The model under review builds one solid part; all positions refer to its coordinate system, in mm. A direction names the side the tool comes from. Give positions to 0.01 mm unless a question says otherwise; leave off trailing zeros. Order: outer loops, then holes, each group sorted by start corner. A loop starts at its lowest first (then second) coordinate and runs counter-clockwise, first axis right, second up.
```python
from build123d import *

# Parameters (mm, degrees)
SKETCH1_W             = 25.4
SKETCH1_H             = 101.6
TOP_DEPTH             = 4.7625
SKETCH2_W             = 25.4
SKETCH2_H             = 101.6
SKETCH2_W_2           = 15.875
SKETCH2_H_2           = 88.9
WALLS_DEPTH           = 31.75
SKETCH9_R             = 3.302
JOINT_HINGE_DEPTH     = 6.35
SKETCH3_R             = 3.175
SHAFT_HOLES_DEPTH     = 23.876
SKETCH13_W            = 1.778
SKETCH13_H            = 5.08
WIRE_LOFT_MOUNT_DEPTH = 12.7
ANTI_FLEX_DEPTH       = 3.175
FILLET1_R             = 2.54
FILLET2_R             = 1.5875


with BuildPart() as part:
    # Sketch1 → Top (new body)
    with BuildSketch(Plane(origin=(0, 0, 0), x_dir=(1, 0, 0), z_dir=(0, 1, 0))):
        Rectangle(SKETCH1_W, SKETCH1_H)
    extrude(amount=TOP_DEPTH)

    # Sketch2 → Walls (add)
    with BuildSketch(Plane(origin=(0, 4.7625, 0), x_dir=(1, 0, 0), z_dir=(0, 1, 0))):
        Rectangle(SKETCH2_W, SKETCH2_H)
        Rectangle(SKETCH2_W_2, SKETCH2_H_2, mode=Mode.SUBTRACT)
    extrude(amount=-WALLS_DEPTH)

    # Sketch9 → Joint Hinge (add)
    with BuildSketch(Plane(origin=(0, 0, 50.8), x_dir=(-1, 0, 0), z_dir=(0, 0, -1))):
        with BuildLine():
            Line((-28.956, 4.7625), (-12.7, 4.7625))
            Line((-12.7, 4.7625), (-12.7, -26.9875))
            Line((-12.7, -26.9875), (-14.756968343, -26.9875))
            ThreePointArc((-14.756968343, -26.9875), (-46.346191201, -22.064629933), (-28.956, 4.7625))
        make_face()
        with Locations((-28.956, -14.2875)):
            Circle(SKETCH9_R, mode=Mode.SUBTRACT)
    extrude(amount=JOINT_HINGE_DEPTH)

    # Sketch3 → Shaft holes (cut)
    with BuildSketch(Plane.ZY.offset(12.7)):
        with Locations((38.1, -11.1125)):
            Circle(SKETCH3_R)
        with BuildLine():
            Line((-25.601638938, -12.7), (-23.061638938, -12.7))
            Line((-23.061638938, -12.7), (-23.061638938, -9.525))
            Line((-23.061638938, -9.525), (-25.601638938, -9.525))
            ThreePointArc((-25.601638938, -9.525), (-38.1, -11.1125), (-25.601638938, -12.7))
        make_face()
    extrude(amount=-SHAFT_HOLES_DEPTH, mode=Mode.SUBTRACT)

    # Sketch13 → Wire Loft Mount (cut)
    with BuildSketch(Plane.XZ):
        with Locations((-2.286, 29.21)):
            Rectangle(SKETCH13_W, SKETCH13_H)
    extrude(amount=-WIRE_LOFT_MOUNT_DEPTH, mode=Mode.SUBTRACT)

    # Sketch15 → Anti-flex (add)
    with BuildSketch(Plane(origin=(0, 4.7625, 0), x_dir=(1, 0, 0), z_dir=(0, 1, 0))):
        Polygon((12.7, -44.45), (28.956, -44.45), (12.7, -28.194), align=None)
        Polygon((12.7, 28.194), (28.956, 44.45), (28.956, 50.8), (12.7, 50.8), align=None)
    extrude(amount=-ANTI_FLEX_DEPTH)

    # Fillet1
    fillet1_edges = [part.edges().sort_by_distance(p)[0] for p in [
        (8.128, 4.7625, -50.8),
        (0, -26.9875, -50.8),
        (1.028484171, -26.9875, 50.8),
        (46.346191201, -22.064629933, 50.8),
        (8.128, 4.7625, 50.8),
    ]]
    fillet(fillet1_edges, radius=FILLET1_R)

    # Fillet2
    # the kernel refuses this fillet: 1.5875 mm, written as the material it takes off along each edge
    with BuildSketch(Plane(origin=(9.893669962, 1.5875, -25.387669962), x_dir=(-0.7071067811865515, 0, -0.7071067811865436), z_dir=(0.7071067811865437, 0, -0.7071067811865515))) as fillet2_piece_1_section:
        with BuildLine():
            CenterArc((FILLET2_R, FILLET2_R), FILLET2_R, 180, 90)
            Line((0, FILLET2_R), (0, 0))
            Line((0, 0), (FILLET2_R, 0))
        make_face()
    fillet2_piece_1 = extrude(amount=30.92695567, mode=Mode.PRIVATE)
    fillet2_piece_1 = split(fillet2_piece_1, bisect_by=Plane(origin=(12.7, 1.942096603, -36.823475324), z_dir=(1, 0, 0)), keep=Keep.TOP, mode=Mode.PRIVATE)
    add(fillet2_piece_1, mode=Mode.SUBTRACT)
    with BuildSketch(Plane(origin=(9.893669962, 4.7625, -25.387669962), x_dir=(-0.7071067811865515, 0, -0.7071067811865436), z_dir=(0.7071067811865437, 0, -0.7071067811865515))) as fillet2_piece_2_section:
        with BuildLine():
            CenterArc((FILLET2_R, -FILLET2_R), FILLET2_R, 90, 90)
            Line((0, -FILLET2_R), (0, 0))
            Line((0, 0), (FILLET2_R, 0))
        make_face()
    fillet2_piece_2 = extrude(amount=30.92695567, mode=Mode.PRIVATE)
    fillet2_piece_2 = split(fillet2_piece_2, bisect_by=Plane(origin=(12.7, 4.407903397, -36.823475324), z_dir=(1, 0, 0)), keep=Keep.TOP, mode=Mode.PRIVATE)
    add(fillet2_piece_2, mode=Mode.SUBTRACT)
    with BuildSketch(Plane(origin=(31.762330038, 1.5875, 47.256330038), x_dir=(-0.7071067811865436, 0, 0.7071067811865515), z_dir=(-0.7071067811865515, 0, -0.7071067811865436))) as fillet2_piece_3_section:
        with BuildLine():
            CenterArc((FILLET2_R, FILLET2_R), FILLET2_R, 180, 90)
            Line((0, FILLET2_R), (0, 0))
            Line((0, 0), (FILLET2_R, 0))
        make_face()
    fillet2_piece_3 = extrude(amount=30.92695567, mode=Mode.PRIVATE)
    fillet2_piece_3 = split(fillet2_piece_3, bisect_by=Plane(origin=(12.7, 1.946775649, 36.567113542), z_dir=(1, 0, 0)), keep=Keep.TOP, mode=Mode.PRIVATE)
    fillet2_piece_3 = split(fillet2_piece_3, bisect_by=Plane(origin=(20.582886458, 1.946775649, 44.45), z_dir=(0, 0, -1)), keep=Keep.TOP, mode=Mode.PRIVATE)
    add(fillet2_piece_3, mode=Mode.SUBTRACT)
    with BuildSketch(Plane(origin=(31.762330038, 4.7625, 47.256330038), x_dir=(-0.7071067811865436, 0, 0.7071067811865515), z_dir=(-0.7071067811865515, 0, -0.7071067811865436))) as fillet2_piece_4_section:
        with BuildLine():
            CenterArc((FILLET2_R, -FILLET2_R), FILLET2_R, 90, 90)
            Line((0, -FILLET2_R), (0, 0))
            Line((0, 0), (FILLET2_R, 0))
        make_face()
    fillet2_piece_4 = extrude(amount=30.92695567, mode=Mode.PRIVATE)
    fillet2_piece_4 = split(fillet2_piece_4, bisect_by=Plane(origin=(12.7, 4.227310256, 42.469450936), z_dir=(1, 0, 0)), keep=Keep.TOP, mode=Mode.PRIVATE)
    fillet2_piece_4 = split(fillet2_piece_4, bisect_by=Plane(origin=(26.668449599, 4.227310256, 44.45), z_dir=(0, 0, -1)), keep=Keep.TOP, mode=Mode.PRIVATE)
    add(fillet2_piece_4, mode=Mode.SUBTRACT)
    with BuildSketch(Plane(origin=(31.762330038, 4.7625, 47.256330038), x_dir=(-0.7071067811865436, 0, 0.7071067811865515), z_dir=(-0.7071067811865515, 0, -0.7071067811865436))) as fillet2_piece_5_section:
        with BuildLine():
            CenterArc((FILLET2_R, -FILLET2_R), FILLET2_R, 90, 90)
            Line((0, -FILLET2_R), (0, 0))
            Line((0, 0), (FILLET2_R, 0))
        make_face()
    fillet2_piece_5 = extrude(amount=30.92695567, mode=Mode.PRIVATE)
    fillet2_piece_5 = split(fillet2_piece_5, bisect_by=Plane(origin=(27.86835314, 4.749091996, 44.45), z_dir=(0, 0, 1)), keep=Keep.TOP, mode=Mode.PRIVATE)
    fillet2_piece_5 = fillet2_piece_5 - Plane(origin=(28.956, -14.2875, 44.898632057), x_dir=(-0.7453559924999297, -0.6666666666666669, 0), z_dir=(0, 0, 1)) * Cylinder(19.05, 69, mode=Mode.PRIVATE)
    add(fillet2_piece_5, mode=Mode.SUBTRACT)


solid = part.part
```
Item 1: For line 1 (X direction, y = -23, z = -6.5); line 2 (Y direction, x = -10, z = 38); line 3 (Y direction, x = 16, z = -36.5), list the stretches that pass through material, from the lowest coordinate up.
Values found:
line 1: x = -12.7 to -7.94, 7.94 to 12.7
line 2: y = -26.99 to -14.29, -7.94 to 4.76
line 3: y = 1.59 to 4.76
Item 2: Take a section at A-A (z = 13.5). Give the boundary of the cut face in (x, y), and give its area (3 significant figures).
Values found:
outline: (-12.7, -26.99) - (-7.94, -26.99) - (-7.94, 0) - (7.94, 0) - (7.94, -26.99) - (12.7, -26.99) - (12.7, 4.76) - (-12.7, 4.76) - close
area: 378 mm2
Item 3: Take a section at B-B (x = 9.5). Give the number of separate pieces and of enclosed holes in the cut face, and give its area (3 significant figures).
Values found:
separate pieces: 1
enclosed holes: 2
area: 3,050 mm2
Item 4: Draft analysis for pull direction X (two halves, no side actions). For faces 1 (the flat face through (28.956, 3, -48)), 2 (the cylindrical face through (1.8, -26.3, 50)), 3 (the flat face through (0, -13, -44.45)), state which applies: released by +X, released by -X, zero draft, split by the parting line, or undercut.
Values found:
face 1: released by +X
face 2: zero draft
face 3: undercut
Item 5: For faces 4 (the flat face through (10, -9.525, -24)), 5 (the flat face through (0, -13, 44.45)), 6 (the flat face through (-3.175, 2, 29)), list the 3-axis set-ups (+Z, -Z, +X, -X, +Y, -Y) from which the entire face can be reached by the end or side of a thin tool; tool diameter is ignored.
Values found:
face 4: -X
face 5: -Y
face 6: +Y, -Y
Item 6: Clearance check with flat-ended pins moving along their axes: pin 1 Ø12 at (x, y) = (21, -6.5) entering from -Z; pin 2 Ø1.9 at (y, z) = (-10, 36.5) entering from -X; pin 3 Ø5 at (x, z) = (-3, 4) entering from -Y. State where each tip first meets the part, or that it passes through.
Values found:
pin 1: stops at z = 44.45
pin 2: stops at x = 11.18
pin 3: stops at y = 0
